Geometry: final body of the model. Coordinates: model frame, mm. A direction names the side the tool comes from. Coordinates: 2 decimals unless noted, no trailing zeros. Write each loop counter-clockwise with the first axis right and the second up, starting at its lowest first coordinate (ties: lowest second). Pieces come first, ordered by that corner, then holes. Notation, with made-up numbers: (69, 69.5) - (73, 69.5) arc R31 cw to (73, 96.5) - close; hole circle Ø9 at (81.25, 41). An arc over 180 degrees is marked (long way). Answer as a JSON object with one key per item and string values. Group by question number.
Item 1: Line query: line 1 along X through (y, z) = (-106, 1.65); line 2 along Z through (x, y) = (16.5, -109.25); line 3 along X through (y, z) = (-107.75, 22.5). Output: solid intervals per line, ascending. Write a range as from..to.
Item 2: First-contact query: pin 1 Ø4 at (y, z) = (-106, 17.5) entering from +X; pin 2 Ø2.5 at (y, z) = (-106, 39) entering from -X. Flat tips, straight axial feed; report the tip coordinate or a pass-through.
Item 3: Section D-D on z = 54. Return loops of the section in (x, y).
Item 4: Section B-B on z = 29. Return loops of the section in (x, y).
Item 5: Set-up query: faces 4 (the flat face through (7.968, -106, 29)), 5 (the cylindrical face through (-18.773, -104.513, 2.535)), 6 (the flat face through (-17, -106, 53)). Return all of +Z, -Z, +X, -X, +Y, -Y with unobstructed straight access to the full face (end or side cutting, diameter ignored); none if empty.
Item 6: Mould query, pull axis Z, two halves, no side actions, for faces 1 (the cylindrical face through (-8.823, -106.056, 5.902)), 2 (the flat face through (-24.968, -106, 55)), 3 (the flat face through (0, -106, 58)). Classes: pulls with the +Z half, pulls with the -Z half, needs draft (parallel to the pull), parting line crosses it, or undercut.
Item 7: Section A-A on y = -106. State how many separate pieces and enclosed holes the cut face has, and give its area (3 significant figures).
Item 8: Section C-C on x = 0. Return loops of the section in (y, z), and give its area (3 significant figures).
```python
from build123d import *

# Parameters (mm, degrees)
SKETCH_1_W               = 49.93556627
SKETCH_1_H               = 8
EXTRUDE_1_DEPTH          = 58
CUT_EXTRUDE_1_DEPTH      = 56
CUT_EXTRUDE_2_DEPTH      = 66
CUT_EXTRUDE_2_DEPTH_BACK = 10
SKETCH_4_R               = 1.5
SKETCH_3_R               = 2.5
CUT_EXTRUDE_3_DEPTH      = 8


with BuildPart() as part:
    # 草图1 → 凸台-拉伸1 (new body)
    with BuildSketch(Plane.XY):
        with Locations((0, -106)):
            Rectangle(SKETCH_1_W, SKETCH_1_H)
    extrude(amount=EXTRUDE_1_DEPTH)

    # 草图2 → 切除-拉伸1 (cut)
    with BuildSketch(Plane.XZ.offset(110)):
        with BuildLine():
            Line((-24.967783135, 53), (-10.967783135, 53))
            ThreePointArc((-10.967783135, 53), (-8.846462792, 52.121320344), (-7.967783135, 50))
            Line((-7.967783135, 50), (-7.967783135, 8))
            ThreePointArc((-7.967783135, 8), (-8.846462792, 5.878679656), (-10.967783135, 5))
            Line((-10.967783135, 5), (-24.967783135, 5))
            Line((-24.967783135, 5), (-24.967783135, 53))
        make_face()
        with BuildLine():
            Line((24.967783135, 5), (10.967783135, 5))
            ThreePointArc((10.967783135, 5), (8.846462792, 5.878679656), (7.967783135, 8))
            Line((7.967783135, 8), (7.967783135, 50))
            ThreePointArc((7.967783135, 50), (8.846462792, 52.121320344), (10.967783135, 53))
            Line((10.967783135, 53), (24.967783135, 53))
            Line((24.967783135, 53), (24.967783135, 5))
        make_face()
    extrude(amount=-CUT_EXTRUDE_1_DEPTH, mode=Mode.SUBTRACT)

    # 草图4 → 切除-拉伸2 (cut, two sides: drawn at the far end of the back side and taken through both)
    with BuildSketch(Plane(origin=(0, 0, 53), x_dir=(-1, 0, 0), z_dir=(0, 0, -1)).offset(-CUT_EXTRUDE_2_DEPTH_BACK)):
        with Locations((18.967783135, -106)):
            Circle(SKETCH_4_R)
        with Locations(Location((-18.967783135, -106, 0), (0, 0, 180))):
            Circle(SKETCH_4_R)
    extrude(amount=CUT_EXTRUDE_2_DEPTH + CUT_EXTRUDE_2_DEPTH_BACK, mode=Mode.SUBTRACT)

    # 草图3 → 切除-拉伸3 (cut)
    with BuildSketch(Plane.XZ.offset(110)):
        with Locations(Location((0, 29, 0), (0, 0, 270))):
            Circle(SKETCH_3_R)
    extrude(amount=-CUT_EXTRUDE_3_DEPTH, mode=Mode.SUBTRACT)


solid = part.part
```
Checks:
{
 "1": {"line 1": "-24.97..-20.47, -17.47..17.47, 20.47..24.97", "line 2": "0..5, 53..58", "line 3": "-7.97..7.97"},
 "2": {"pin 1": "x = 7.97", "pin 2": "x = -7.97"},
 "3": {"outline": "(-24.97, -110) - (24.97, -110) - (24.97, -102) - (-24.97, -102) - close; hole circle Ø3 at (-18.97, -106); hole circle Ø3 at (18.97, -106)"},
 "4": {"outline": "(-7.97, -110) - (-2.5, -110) - (-2.5, -102) - (-7.97, -102) - close; (2.5, -110) - (7.97, -110) - (7.97, -102) - (2.5, -102) - close"},
 "5": {"face 4": "+X, +Y, -Y", "face 5": "+Z, -Z", "face 6": "-X, +Y, -Y"},
 "6": {"face 1": "undercut", "face 2": "needs draft", "face 3": "pulls with the +Z half"},
 "7": {"separate pieces": "5", "enclosed holes": "1", "area": "1,190 mm^2"},
 "8": {"outline": "(-110, 0) - (-102, 0) - (-102, 26.5) - (-110, 26.5) - close; (-110, 31.5) - (-102, 31.5) - (-102, 58) - (-110, 58) - close", "area": "424 mm^2"}
}
